Check sheet for the modelled part. Datum: model origin and axes. Units: mm. Face numbers are marked on the shaded views. A direction names the side the tool comes from. Coordinates: 2 decimals unless noted, no trailing zeros. Loops run counter-clockwise (first coordinate to the right, second up) from the corner with the lowest first, then second, coordinate; pieces in that order, holes last. Notation, with made-up numbers: M -7.75,73 L 38.25,73 A8 ccw 38.25,84 Z; hole C 21.25,-37.5 d6. An arc over 180 degrees is marked long. Use CSV: the item, a comma, the result in double quotes. Start each with the question number.
(1) Section check D-D on x = 37. Record the cut outline in (y, z).
(2) Go/stop test with flat-tipped pins: pin 1 Ø12.5 at (x, y) = (14.5, -13) entering from -Z; pin 2 Ø6.5 at (x, z) = (-20, -27) entering from +Y; pin 3 Ø7.5 at (x, y) = (16, -8) entering from +Z. Record where each tip stops, or that it passes through.
(3) Section check A-A on z = 27.5. Record the cut outline in (x, y), and give its area (3 significant figures).
(4) Scan lines: line 1 (X direction, y = -23.1, z = -27.5); line 2 (Z direction, x = 23, y = -5.25); line 3 (Z direction, x = -38.5, y = -22.5). Record each from-to range of solid material in increasing order.
(5) Set-up check for the marked faces 4, 5 and 6: record each of +Z, -Z, +X, -X, +Y, -Y from which the full face is reachable in a straight line by a thin tool's end or side.
(6) Section check C-C on y = -12.25. Record the cut outline in (x, z).
(7) Draft check along Z on the marked faces 1, 2 and 3. Enter one of: pulls with the +Z half, pulls with the -Z half, needs draft (parallel to the pull), parting line crosses it, or undercut.
(8) Section check B-B on x = -33.5. Record the cut outline in (y, z).
from build123d import *

# Parameters (mm, degrees)
SKETCH1_W           = 99
SKETCH1_H           = 43
SKETCH1_H_2         = 2
BOSS_EXTRUDE1_DEPTH = 3
SKETCH1_5_W         = 99
SKETCH1_5_H         = 2
BOSS_EXTRUDE2_DEPTH = 25
SKETCH3_W           = 99
SKETCH3_H           = 8
SKETCH3_R           = 1.6
BOSS_EXTRUDE3_DEPTH = 3


with BuildPart() as part:
    # Sketch1 → Boss-Extrude1 (new body)
    with BuildSketch(Plane(origin=(0, 0, 0), x_dir=(1, 0, 0), z_dir=(0, 1, 0))):
        Rectangle(SKETCH1_W, SKETCH1_H)
        with Locations((0, -22.5)):
            Rectangle(SKETCH1_W, SKETCH1_H_2)
        with Locations((0, 22.5)):
            Rectangle(SKETCH1_W, SKETCH1_H_2)
    extrude(amount=BOSS_EXTRUDE1_DEPTH)

    # Sketch1_5 → Boss-Extrude2 (add)
    with BuildSketch(Plane(origin=(0, 0, 0), x_dir=(1, 0, 0), z_dir=(0, 1, 0))):
        with Locations((0, -22.5)):
            Rectangle(SKETCH1_5_W, SKETCH1_5_H)
        with Locations((0, 22.5)):
            Rectangle(SKETCH1_5_W, SKETCH1_5_H)
    extrude(amount=-BOSS_EXTRUDE2_DEPTH)

    # Sketch3 → Boss-Extrude3 (add)
    # profile 1 of 2: a face of its own
    with BuildSketch(Plane.XZ.offset(25)):
        with Locations((0, 27.5)):
            Rectangle(SKETCH3_W, SKETCH3_H)
        with Locations(Location((-33.5, 27.5, 0), (0, 0, 270))):
            Circle(SKETCH3_R, mode=Mode.SUBTRACT)
        with Locations(Location((33.5, 27.5, 0), (0, 0, 90))):
            Circle(SKETCH3_R, mode=Mode.SUBTRACT)
    # profile 2 of 2: a face of its own
    with BuildSketch(Plane.XZ.offset(25)):
        with Locations((0, -27.5)):
            Rectangle(SKETCH3_W, SKETCH3_H)
        with Locations(Location((33.5, -27.5, 0), (0, 0, 270))):
            Circle(SKETCH3_R, mode=Mode.SUBTRACT)
        with Locations(Location((-33.5, -27.5, 0), (0, 0, 90))):
            Circle(SKETCH3_R, mode=Mode.SUBTRACT)
    extrude(amount=-BOSS_EXTRUDE3_DEPTH)


solid = part.part
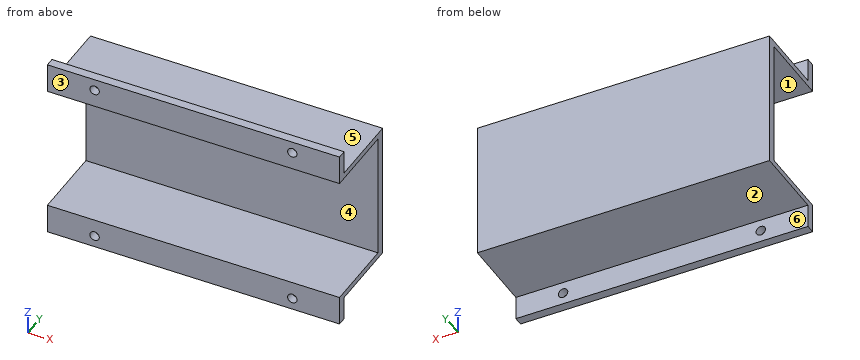
Outcome:
1,outline,"M -25,-31.5 L -22,-31.5 L -22,-23.5 L 3,-23.5 L 3,23.5 L -22,23.5 L -22,31.5 L -25,31.5 L -25,21.5 L 0,21.5 L 0,-21.5 L -25,-21.5 Z"
2,pin 1,"stops at z = -23.5"
2,pin 2,"stops at y = -22"
2,pin 3,"stops at z = 23.5"
3,outline,"M -49.5,-25 L -35.1,-25 L -35.1,-22 L -49.5,-22 Z; M -31.9,-25 L 31.9,-25 L 31.9,-22 L -31.9,-22 Z; M 35.1,-25 L 49.5,-25 L 49.5,-22 L 35.1,-22 Z"
3,area,"278 mm²"
4,line 1,"x = -49.5 to -35.1, -31.9 to 31.9, 35.1 to 49.5"
4,line 2,"z = -23.5 to -21.5, 21.5 to 23.5"
4,line 3,"z = -31.5 to -21.5, 21.5 to 31.5"
5,face 4,"+X, -X, -Y"
5,face 5,"+Z, +X, -X, +Y"
5,face 6,"-Z, +X, -X, +Y"
6,outline,"M -49.5,-23.5 L 49.5,-23.5 L 49.5,-21.5 L -49.5,-21.5 Z; M -49.5,21.5 L 49.5,21.5 L 49.5,23.5 L -49.5,23.5 Z"
7,face 1,"undercut"
7,face 2,"pulls with the -Z half"
7,face 3,"needs draft"
8,outline,"M -25,-31.5 L -22,-31.5 L -22,-29.1 L -25,-29.1 Z; M -25,-25.9 L -22,-25.9 L -22,-23.5 L 3,-23.5 L 3,23.5 L -22,23.5 L -22,25.9 L -25,25.9 L -25,21.5 L 0,21.5 L 0,-21.5 L -25,-21.5 Z; M -25,29.1 L -22,29.1 L -22,31.5 L -25,31.5 Z"
